Read the model definition and answer for the solid it produces. Units are mm, in the model's axes. Face numbers are marked on the shaded views. A direction names the side the tool comes from. Coordinates: 2 decimals unless noted, no trailing zeros. Order: outer loops, then holes, each group sorted by start corner. A loop starts at its lowest first (then second) coordinate and runs counter-clockwise, first axis right, second up. Notation, with made-up numbers: (89.5, 67.25) -> (125.5, 67.25) arc R34 ccw to (125.5, 99.25) -> close; hole circle Ø7 at (46, 11.25). An arc over 180 degrees is marked (long way). Answer in a Markdown table with one row per item.
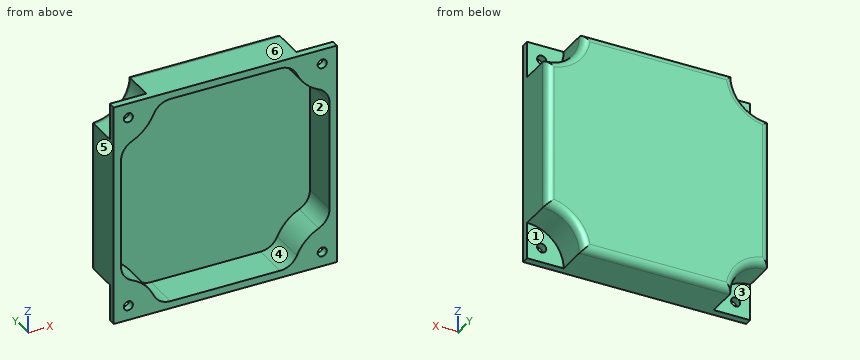
from build123d import *

# Parameters (mm, degrees)
SKETCH2_W           = 61
SKETCH2_H           = 61
BOSS_EXTRUDE1_DEPTH = 12
SKETCH4_R           = 10
CUT_EXTRUDE3_DEPTH  = 10
CUT_EXTRUDE5_DEPTH  = 10
FILLET2_R           = 2
FILLET3_R           = 5


with BuildPart() as part:
    # Sketch2 → Boss-Extrude1 (new body)
    with BuildSketch(Plane(origin=(0, 0, 0), x_dir=(1, 0, 0), z_dir=(0, 1, 0))):
        Rectangle(SKETCH2_W, SKETCH2_H)
    extrude(amount=BOSS_EXTRUDE1_DEPTH)

    # Sketch4 → Cut-Extrude3 (cut)
    with BuildSketch(Plane(origin=(0, 12, 0), x_dir=(1, 0, 0), z_dir=(0, 1, 0))):
        with Locations((30.5, -30.5)):
            Circle(SKETCH4_R)
        with Locations((-30.5, -30.5)):
            Circle(SKETCH4_R)
        with Locations((-30.5, 30.5)):
            Circle(SKETCH4_R)
        with Locations((30.5, 30.5)):
            Circle(SKETCH4_R)
    extrude(amount=-CUT_EXTRUDE3_DEPTH, mode=Mode.SUBTRACT)

    # Sketch8 → Cut-Extrude5 (cut)
    with BuildSketch(Plane.XZ):
        with BuildLine():
            Line((-18.667840434, -28.5), (18.667840434, -28.5))
            ThreePointArc((18.667840434, -28.5), (22.014718626, -22.014718626), (28.5, -18.667840434))
            Line((28.5, -18.667840434), (28.5, 18.667840434))
            ThreePointArc((28.5, 18.667840434), (22.014718626, 22.014718626), (18.667840434, 28.5))
            Line((18.667840434, 28.5), (-18.667840434, 28.5))
            ThreePointArc((-18.667840434, 28.5), (-22.014718626, 22.014718626), (-28.5, 18.667840434))
            Line((-28.5, 18.667840434), (-28.5, -18.667840434))
            ThreePointArc((-28.5, -18.667840434), (-22.014718626, -22.014718626), (-18.667840434, -28.5))
        make_face()
    extrude(amount=-CUT_EXTRUDE5_DEPTH, mode=Mode.SUBTRACT)

    # Fillet2
    fillet2_edges = [part.edges().sort_by_distance(p)[0] for p in [
        (30.5, 12, 0),
        (0, 12, -30.5),
        (-30.5, 12, 0),
        (0, 12, 30.5),
        (23.428932188, 12, -23.428932188),
        (-23.428932188, 12, -23.428932188),
        (-23.428932188, 12, 23.428932188),
        (23.428932188, 12, 23.428932188),
    ]]
    fillet(fillet2_edges, radius=FILLET2_R)

    # Sketch15 → M3x0.5 Tapped Hole1 (revolve, cut)
    with BuildSketch(Plane(origin=(26.5, 2, 26.5), x_dir=(0, 0, 1), z_dir=(1, 0, 0))):
        Polygon((0, 0), (0, 8.251075774), (1.25, 7.5), (1.25, 0), align=None)
    m3x0_5_tapped_hole1 = revolve(axis=Axis((26.5, 8.35, 26.5), (0, -1, 0)), mode=Mode.SUBTRACT)

    # Mirror1: M3x0.5 Tapped Hole1 across plane
    add(m3x0_5_tapped_hole1.mirror(Plane.XY), mode=Mode.SUBTRACT)

    # Mirror2: M3x0.5 Tapped Hole1 across plane
    add(m3x0_5_tapped_hole1.mirror(Plane(origin=(0, 0, 0), x_dir=(0, 0, 1), z_dir=(1, 0, 0))), mode=Mode.SUBTRACT)

    # Mirror2 copy 1 sketch → Mirror2 copy 1 (revolve, cut)
    with BuildSketch(Plane(origin=(-26.5, 2, -26.5), x_dir=(0, 0, -1), z_dir=(-1, 0, 0))):
        Polygon((0, 0), (0, 8.251075774), (1.25, 7.5), (1.25, 0), align=None)
    revolve(axis=Axis((-26.5, 8.35, -26.5), (0, -1, 0)), mode=Mode.SUBTRACT)

    # Fillet3
    fillet3_edges = [part.edges().sort_by_distance(p)[0] for p in [
        (28.5, 5, -18.667840434),
        (18.667840434, 5, -28.5),
        (-18.667840434, 5, -28.5),
        (-28.5, 5, -18.667840434),
        (-28.5, 5, 18.667840434),
        (-18.667840434, 5, 28.5),
        (18.667840434, 5, 28.5),
        (28.5, 5, 18.667840434),
    ]]
    fillet(fillet3_edges, radius=FILLET3_R)


solid = part.part
Q1. For the marked faces 1, 2 and 3, determine the directions among +Z, -Z, +X, -X, +Y, -Y from which every point of the face is accessible in a straight line to the end or side of a thin tool.
Outcome:
| item | result |
|---|---|
| face 1 | -Z, +X, +Y |
| face 2 | -Y |
| face 3 | -Z, -X, +Y |
Q2. The part is cut by section B-B (z = -5.5). Write down the section's boundary in (x, y).
Outcome:
| item | result |
|---|---|
| outline | (-30.5, 0) -> (-28.5, 0) -> (-28.5, 10) -> (28.5, 10) -> (28.5, 0) -> (30.5, 0) -> (30.5, 10) arc R2 ccw to (28.5, 12) -> (-28.5, 12) arc R2 ccw to (-30.5, 10) -> close |
Q3. The part is cut by section D-D (x = -26.5). Give the number of separate pieces and of enclosed holes in the cut face, then the cut area to 3 significant figures.
Outcome:
| item | result |
|---|---|
| separate pieces | 3 |
| enclosed holes | 0 |
| area | 157 mm² |
Q4. The part is cut by section A-A (y = 6.5). Write down the section's boundary in (x, z), then the cut area to 3 significant figures.
Outcome:
| item | result |
|---|---|
| outline | (-30.5, -20.5) arc R10 cw to (-20.5, -30.5) -> (20.5, -30.5) arc R10 cw to (30.5, -20.5) -> (30.5, 20.5) arc R10 cw to (20.5, 30.5) -> (-20.5, 30.5) arc R10 cw to (-30.5, 20.5) -> close; hole (-28.5, -15.01) arc R5 ccw to (-25.56, -19.56) arc R12 cw to (-19.56, -25.56) arc R5 ccw to (-15.01, -28.5) -> (15.01, -28.5) arc R5 ccw to (19.56, -25.56) arc R12 cw to (25.56, -19.56) arc R5 ccw to (28.5, -15.01) -> (28.5, 15.01) arc R5 ccw to (25.56, 19.56) arc R12 cw to (19.56, 25.56) arc R5 ccw to (15.01, 28.5) -> (-15.01, 28.5) arc R5 ccw to (-19.56, 25.56) arc R12 cw to (-25.56, 19.56) arc R5 ccw to (-28.5, 15.01) -> close |
| area | 453 mm² |
Q5. Consider line 1 (Z direction, x = 26.5, y = 1.25); line 2 (X direction, y = 9.5, z = 2). Determine where each line is inside the solid, lowest interval first.
Outcome:
| item | result |
|---|---|
| line 1 | -30.5 to -27.75, -25.25 to -19.01, 19.01 to 25.25, 27.75 to 30.5 |
| line 2 | -30.5 to -28.5, 28.5 to 30.5 |
Q6. Given pin 1 (3 mm diameter, centred on x = -24.5, z = 27, fed in from +Y); pin 2 (3 mm diameter, centred on x = 23.5, z = 24, fed in from +Y); pin 3 (4 mm diameter, centred on x = 5.5, z = -4.5, fed in from -Y), each flat-ended and moving along its own axis, determine where each tip first touches the part or whether it passes through.
Outcome:
| item | result |
|---|---|
| pin 1 | y = 2 |
| pin 2 | y = 11.76 |
| pin 3 | y = 10 |
Q7. For a pull along Z with two mould halves and no side action, classify the marked faces 4, 5 and 6 as pulls with the +Z half, pulls with the -Z half, needs draft (parallel to the pull), parting line crosses it, or undercut.
Outcome:
| item | result |
|---|---|
| face 4 | undercut |
| face 5 | needs draft |
| face 6 | pulls with the +Z half |
Q8. The part is cut by section C-C (x = 7.5). Write down the section's boundary in (y, z).
Outcome:
| item | result |
|---|---|
| outline | (0, -30.5) -> (10, -30.5) arc R2 ccw to (12, -28.5) -> (12, 28.5) arc R2 ccw to (10, 30.5) -> (0, 30.5) -> (0, 28.5) -> (10, 28.5) -> (10, -28.5) -> (0, -28.5) -> close |
